Design review of the part built by this model. Coordinates are the model's own, in mm. Face numbers are marked on the shaded views. A direction names the side the tool comes from. Coordinates: 2 decimals unless noted, no trailing zeros. Write each loop counter-clockwise with the first axis right and the second up, starting at its lowest first coordinate (ties: lowest second). Pieces come first, ordered by that corner, then holes.
Q1. Take a section at D-D, the plane x = -3.25. Write out the cut boundary in (y, z), plus the area to 4 significant figures.
Q2. Take a section at B-B, the plane y = 5. Write out the cut boundary in (x, z).
Q3. For L1, parallel to X at y = 7, z = -51.75; L2, parallel to X at y = 4, z = 2.5; L3, parallel to Z at x = 2.75, y = 5, list the stretches that pass through material, from the lowest coordinate up.
Q4. For the marked faces 1 and 2, list the 3-axis set-ups (+Z, -Z, +X, -X, +Y, -Y) from which the entire face can be reached by the end or side of a thin tool; tool diameter is ignored.
Q5. Take a section at C-C, the plane z = -51.75. Write out the cut boundary in (x, y).
Q6. Take a section at A-A, the plane x = 3.25. Write out the cut boundary in (y, z).
Q7. For pin 1 Ø1.5 at (x, z) = (-2.5, -50.5) entering from +Y; pin 2 Ø2 at (x, z) = (3.25, -58.25) entering from -Y; pin 3 Ø4 at (y, z) = (5, 4) entering from -X; pin 4 Ø7.5 at (x, y) = (1.5, 64.5) entering from +Z, all flat-tipped, find the tip position at first contact; note any pin that passes through.
Autodesk Inventor part; units mm, degrees
ref_plane "YZ Plane" through (0, 0, 0) normal (1, 0, 0) x (0, 1, 0)
ref_plane "XZ Plane" through (0, 0, 0) normal (0, 1, 0) x (-1, 0, 0)
ref_plane "XY Plane" through (0, 0, 0) normal (0, 0, 1) x (1, 0, 0)
sketch "Boceto2" plane through (0, 0, 0) normal (0, 1, 0) x (-1, 0, 0)
  line L0 (7.5, 100) -> (-7.5, 100)
  line L1 (-7.5, 100) -> (-7.5, -100)
  line L2 (-7.5, -100) -> (7.5, -100)
  line L3 (7.5, -100) -> (7.5, 100)
  line L4 (7.5, 100) -> (-7.5, -100) construction
  line L5 (-7.5, 100) -> (7.5, -100) construction
  point P0 (0, 0)
  dimension "d7" = 15
  dimension "d8" = 200
extrude "Extrusión1" add sketch "Boceto2" along normal blind 10
sketch "Boceto3" plane through (0, 10, 0) normal (0, 1, 0) x (1, 0, 0)
  circle A0 centre (3.25, 58.25) radius 1.75
  line L0 (5, 50) -> (-5, 50)
  line L1 (-5, 50) -> (-5, 60)
  line L2 (-5, 60) -> (5, 60)
  line L3 (5, 60) -> (5, 50)
  line L4 (5, 50) -> (-5, 60) construction
  line L5 (-5, 50) -> (5, 60) construction
  circle A1 centre (-3.25, 51.75) radius 1.75
  line L6 (7.5, 100) -> (-7.5, 100)
  line L7 (-7.5, 0) -> (3.408, 0)
  line L8 (5, -60) -> (5, -50)
  line L9 (-5, -60) -> (5, -60)
  line L10 (5, -50) -> (-5, -50)
  line L11 (-5, -50) -> (-5, -60)
  line L12 (-5, -50) -> (5, -60) construction
  circle A2 centre (-3.25, -51.75) radius 1.75
  line L13 (5, -50) -> (-5, -60) construction
  circle A3 centre (3.25, -58.25) radius 1.75
  line L14 (-7.5, -100) -> (7.5, -100)
  point P0 (0, 0)
  point P1 (-5, 55)
  point P2 (0, 100)
  point P3 (-5, -55)
  dimension "d11" = 3.5
  dimension "d12" = 1.75
  dimension "d13" = 1.75
  dimension "d14" = 1.75
  dimension "d15" = 1.75
  dimension "d16" = 10
  dimension "d17" = 10
  dimension "d19" = 40
  dimension "d81" = 40
hole "Agujero1" at (3.25, 10, 58.25) at (-3.25, 10, 51.75) at (3.25, 10, -58.25) at (-3.25, 10, -51.75) direction (0, -1, 0) diameter 3.5 end through all
sketch "Boceto4" plane through (0, 10, 0) normal (0, 1, 0) x (1, 0, 0)
  line L0 (-7.5, 100) -> (-7.5, -100)
  line L1 (-7.5, -100) -> (7.5, -100)
  line L2 (7.5, -100) -> (7.5, -80)
  line L3 (7.5, -80) -> (-7.5, -80)
  line L4 (-7.5, -80) -> (-7.5, -100)
  line L5 (-7.5, 0) -> (1.0116, 0)
  line L6 (-7.5, -100) -> (-7.5, 100)
  line L7 (-7.5, 100) -> (7.5, 100)
  line L8 (7.5, 100) -> (7.5, 80)
  line L9 (7.5, 80) -> (-7.5, 80)
  line L10 (-7.5, 80) -> (-7.5, 100)
  point P0 (0, 0)
  point P1 (-7.5, -80)
  point P2 (-7.5, 80)
  dimension "d27" = 15
  dimension "d28" = 20
extrude "Extrusión2" add sketch "Boceto4" along normal blind 80
sketch "Boceto5" plane through (0, 90, 0) normal (0, 1, 0) x (1, 0, 0)
  line L0 (-7.5, -100) -> (7.5, -100)
  line L1 (-7.5, -100) -> (49.5, -100)
  line L2 (49.5, -100) -> (49.5, 100)
  line L3 (49.5, 100) -> (-7.5, 100)
  line L4 (-7.5, 100) -> (-7.5, -100)
  line L5 (49.5, -100) -> (-150.5, -100)
  line L6 (-150.5, -100) -> (-150.5, 100)
  line L7 (-150.5, 100) -> (49.5, 100)
  line L8 (49.5, 100) -> (49.5, -100)
  point P0 (0, 0)
  point P1 (-7.5, 100)
  dimension "d31" = 57
  dimension "d32" = 200
  dimension "d75" = 200
extrude "Extrusión3" add sketch "Boceto5" along normal blind 110
sketch "Boceto6" plane through (0, 200, 0) normal (0, 1, 0) x (1, 0, 0)
  line L0 (49.5, 100) -> (7.5, 100)
  line L1 (49.5, 100) -> (29.5, 100)
  line L2 (29.5, 100) -> (29.5, 80)
  line L3 (7.5, -100) -> (49.5, -100)
  line L4 (28.5, -100) -> (28.5, -80)
  line L5 (-150.5, 100) -> (-150.5, -100)
  line L6 (29.5, 80) -> (-150.5, 80)
  line L7 (-150.5, 80) -> (-150.5, -80)
  line L8 (-150.5, -80) -> (29.5, -80)
  line L9 (29.5, -80) -> (29.5, 80)
  line L10 (-150.5, -100) -> (49.5, -100)
  point P0 (7.5, 80)
  point P1 (-50.5, -100)
  dimension "d36" = 20
  dimension "d37" = 20
  dimension "d38" = 20
  dimension "d77" = 20
extrude "Extrusión4" cut sketch "Boceto6" against normal blind 90 contours L8 L5 L6 L9
sketch "Boceto7" plane through (-150.5, 90, -100) normal (-1, 0, 0) x (0, 0, 1)
  line L0 (0, 110) -> (20, 110)
  line L1 (20, 110) -> (10, 110)
  line L2 (10, 110) -> (10, 20)
  line L3 (10, 20) -> (20, 20)
  line L4 (20, 20) -> (20, 110)
  line L5 (180, 110) -> (180, 20)
  line L6 (180, 110) -> (190, 110)
  line L7 (190, 110) -> (190, 20)
  line L8 (190, 20) -> (180, 20)
  line L9 (180, 20) -> (180, 110)
  line L10 (200, 0) -> (200, 110)
  line L11 (0, 0) -> (0, 110)
  line L12 (0, 110) -> (10, 110)
  line L13 (10, 110) -> (10, 20)
  line L14 (10, 20) -> (0, 20)
  line L15 (0, 20) -> (0, 110)
  line L16 (200, 110) -> (0, 110)
  line L17 (200, 110) -> (190, 110)
  line L18 (190, 110) -> (190, 20)
  line L19 (190, 20) -> (200, 20)
  line L20 (200, 20) -> (200, 110)
  point P0 (100, -90)
  dimension "d63" = 10
  dimension "d65" = 10
  dimension "d76" = 10
extrude "Extrusión5" cut sketch "Boceto7" against normal blind 30 contours L0 L4 L3 L2 | L6 L7 L8 L5
sketch "Boceto8" plane through (-7.5, 0, 100) normal (0, 0, 1) x (1, 0, 0)
  line L0 (-113, 110) -> (-113, 200)
  line L1 (-113, 200) -> (-113, 110)
  circle A0 centre (-124.75, 183.25) radius 1.75
  line L2 (-123, 175) -> (-133, 175)
  line L3 (-133, 175) -> (-133, 185)
  line L4 (-133, 185) -> (-123, 185)
  line L5 (-123, 185) -> (-123, 175)
  line L6 (-123, 175) -> (-133, 185) construction
  line L7 (-133, 175) -> (-123, 185) construction
  circle A1 centre (-131.25, 176.75) radius 1.75
  line L8 (-143, 200) -> (57, 200)
  line L9 (-143, 90) -> (-143, 200)
  line L10 (-113, 155) -> (-128, 155)
  line L11 (-123, 125) -> (-123, 135)
  line L12 (-133, 125) -> (-123, 125)
  line L13 (-123, 135) -> (-133, 125) construction
  line L14 (-123, 135) -> (-133, 135)
  line L15 (-133, 135) -> (-123, 125) construction
  circle A2 centre (-131.25, 133.25) radius 1.75
  line L16 (-133, 135) -> (-133, 125)
  circle A3 centre (-124.75, 126.75) radius 1.75
  line L17 (-143, 110) -> (-113, 110)
  point P0 (7.5, 0)
  point P1 (-133, 180)
  point P2 (-123, 180)
  point P3 (-133, 130)
  point P4 (-123, 130)
  dimension "d45" = 3.5
  dimension "d46" = 1.75
  dimension "d47" = 1.75
  dimension "d48" = 1.75
  dimension "d49" = 1.75
  dimension "d50" = 10
  dimension "d51" = 10
  dimension "d52" = 15
  dimension "d53" = 10
  dimension "d54" = 10
  dimension "d55" = 15
hole "Agujero2" at (-132.25, 183.25, 100) at (-138.75, 176.75, 100) at (-138.75, 133.25, 100) at (-132.25, 126.75, 100) direction (0, 0, -1) diameter 3.5 end through all
ref_plane "Plano de trabajo1" through (-150.5, 90, 100) normal (0, -1, 0) x (1, 0, 0)
split "Dividir1" plane through (-150.5, 90, 100) removes the side toward (0, 1, 0)
ref_plane "Plano de trabajo2" through (-7.5, 10, 0) normal (0, 0, 1) x (1, 0, 0)
sketch "Boceto9" plane through (7.5, 0, 100) normal (1, 0, 0) x (0, 0, -1)
  circle A0 centre (96, 5) radius 1.75
  circle A1 centre (104, 5) radius 1.75
  point P0 (100, 0)
  point P1 (100, 0)
  dimension "d89" = 3.5
hole "Agujero3" at (7.5, 5, 4) at (7.5, 5, -4) direction (-1, 0, 0) diameter 3.5 end through all
sketch "Boceto10" plane through (0, 10, 0) normal (0, 1, 0) x (1, 0, 0)
  line L0 (0, 0) -> (0, -10)
  line L1 (0, -10) -> (7.5, -10)
  line L2 (7.5, -80) -> (7.5, 80)
  line L3 (0, 0) -> (0, 10)
  line L4 (0, 10) -> (-7.5, 10)
  line L5 (-7.5, 80) -> (-7.5, -80)
  dimension "d97" = 10
  dimension "d98" = 10
split body "Dividir2" sketch "Boceto10" result one side removed curves L1 L0 L3 L4 removed pieces at (-7, 33.3333, 93.3333)
properties part number "container_front_foot_2"
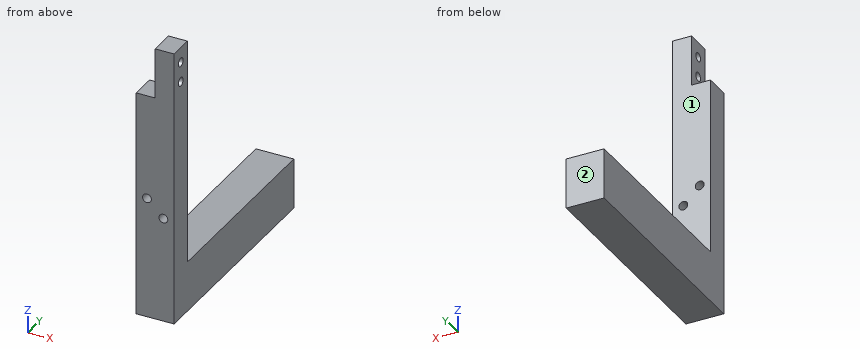
Responses:
1. outline: (0, -100) - (90, -100) - (90, -80) - (10, -80) - (10, -53.5) - (0, -53.5) - close; (0, -50) - (10, -50) - (10, -10) - (0, -10) - close
1. area: 2,465 mm2
2. outline: (-7.5, -100) - (7.5, -100) - (7.5, -5.75) - (0, -5.75) - (0, -10) - (-7.5, -10) - close; (0, -2.25) - (7.5, -2.25) - (7.5, 2.25) - (0, 2.25) - close; (0, 5.75) - (7.5, 5.75) - (7.5, 10) - (0, 10) - close; hole circle Ø3.5 at (-3.25, -51.75); hole circle Ø3.5 at (3.25, -58.25)
3. L1: x = -7.5 to -5, -1.5 to 7.5
3. L2: x = 0 to 7.5
3. L3: z = -100 to -59.93, -56.57 to -5.75, -2.25 to 2.25, 5.75 to 10
4. face 1: +Z, +X, -X, +Y
4. face 2: +Z, -Z, +X, -X, +Y
5. outline: (-7.5, 0) - (-5, 0) - (-5, 10) - (-7.5, 10) - close; (-1.5, 0) - (7.5, 0) - (7.5, 10) - (-1.5, 10) - close
6. outline: (0, -100) - (90, -100) - (90, -80) - (10, -80) - (10, -60) - (0, -60) - close; (0, -56.5) - (10, -56.5) - (10, 10) - (0, 10) - close; hole circle Ø3.5 at (5, -4); hole circle Ø3.5 at (5, 4)
7. pin 1: stops at y = 10
7. pin 2: passes through
7. pin 3: stops at x = 0
7. pin 4: stops at z = -80
